Verification items for the finished model (mm, model axes). Face numbers are marked on the shaded views. A direction names the side the tool comes from. Give positions to 0.01 mm unless a question says otherwise; leave off trailing zeros. Loops run counter-clockwise (first coordinate to the right, second up) from the corner with the lowest first, then second, coordinate; pieces in that order, holes last. Notation, with made-up numbers: (32.5, 49.5) - (89.5, 49.5) arc R12 cw to (89.5, 58.5) - close; hole circle Ø1 at (-31, 50.5). An arc over 180 degrees is marked (long way). Answer in a Markdown table with one row per item.
```python
from build123d import *

# Parameters (mm, degrees)
F0_W     = 508
F0_H     = 762
F0_W_2   = 474.472
F0_H_2   = 736.6
F1_DEPTH = 330.2
F3_DEPTH = 762.001


with BuildPart() as f1:
    # F0 (on Top) → F1 (new body)
    with BuildSketch(Plane.XY):
        with Locations((254, 381)):
            Rectangle(F0_W, F0_H)
        with Locations((254, 381)):
            Rectangle(F0_W_2, F0_H_2, mode=Mode.SUBTRACT)
    extrude(amount=F1_DEPTH)

    # F2 (on Front) → F3 (cut, through all)
    with BuildSketch(Plane.XZ):
        Polygon((0, 330.2), (0, 127), (254, 330.2), align=None)
        Polygon((508, 330.2), (254, 330.2), (508, 127), align=None)
    extrude(amount=-F3_DEPTH, mode=Mode.SUBTRACT)


solid = f1.part
```
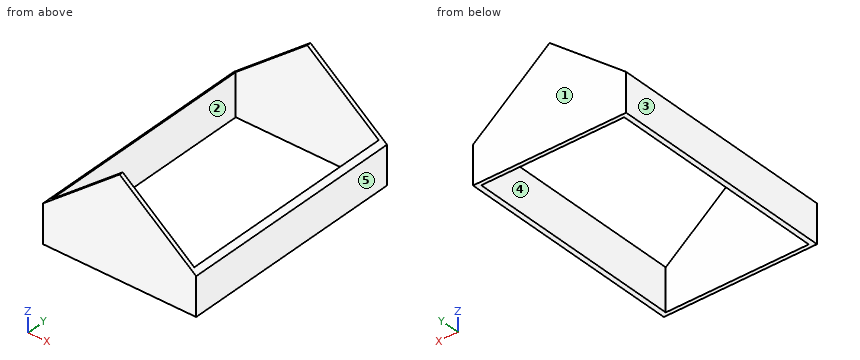
Q1. Sectioned sample at A-A (y = 616). Record the cut outline in (x, z), and give its area (3 significant figures).
Completed:
| item | result |
|---|---|
| outline | (0, 0) - (16.76, 0) - (16.76, 140.41) - (0, 127) - close; (491.24, 0) - (508, 0) - (508, 127) - (491.24, 140.41) - close |
| area | 4,480 mm^2 |
Q2. Sectioned sample at B-B (x = 379.5). Record the cut outline in (y, z).
Completed:
| item | result |
|---|---|
| outline | (0, 0) - (12.7, 0) - (12.7, 229.8) - (0, 229.8) - close; (749.3, 0) - (762, 0) - (762, 229.8) - (749.3, 229.8) - close |
Q3. Thickness scan on line 1 (Y direction, x = 409, z = 199); line 2 (X direction, y = 556, z = 48); line 3 (X direction, y = 540.5, z = 132). Record the ranges inside material, lowest first.
Completed:
| item | result |
|---|---|
| line 1 | 0 to 12.7, 749.3 to 762 |
| line 2 | 0 to 16.76, 491.24 to 508 |
| line 3 | 6.25 to 16.76, 491.24 to 501.75 |
Q4. Sectioned sample at C-C (z = 117). Record the cut outline in (x, y), and give its area (3 significant figures).
Completed:
| item | result |
|---|---|
| outline | (0, 0) - (508, 0) - (508, 762) - (0, 762) - close; hole (16.76, 12.7) - (491.24, 12.7) - (491.24, 749.3) - (16.76, 749.3) - close |
| area | 37,600 mm^2 |
Q5. Tool access check on the marked faces 1 and 2. Record the directions out of +Z, -Z, +X, -X, +Y, -Y that give a thin tool (end or side, any length) a straight path to the whole face; none if there is none.
Completed:
| item | result |
|---|---|
| face 1 | +Z, -Z, +X, -X, +Y |
| face 2 | +Z, -Z |
Q6. Draft check along X on the marked faces 3, 4 and 5. Enter one of: +X half, -X half, draft (parallel to the pull), parting line (faces both ways), or undercut.
Completed:
| item | result |
|---|---|
| face 3 | -X half |
| face 4 | undercut |
| face 5 | +X half |
